```python
from build123d import *

# Parameters (mm, degrees)
SKETCH2_W           = 139.7
SKETCH2_H           = 88.9
BOSS_EXTRUDE1_DEPTH = 5.08
SKETCH3_R           = 1.905
BOSS_EXTRUDE2_DEPTH = 12.7
FILLET1_R           = 5.08
SKETCH4_W           = 25.4
SKETCH4_H           = 25.4
CUT_EXTRUDE1_DEPTH  = 5.08
FILLET2_R           = 5.08


with BuildPart() as part:
    # Sketch2 → Boss-Extrude1 (new body)
    with BuildSketch(Plane(origin=(0, 0, 0), x_dir=(0, 0, -1), z_dir=(1, 0, 0))):
        with Locations((0.114290462, 4.230322371)):
            Rectangle(SKETCH2_W, SKETCH2_H)
    extrude(amount=BOSS_EXTRUDE1_DEPTH)

    # Sketch3 → Boss-Extrude2 (add)
    with BuildSketch(Plane.ZY):
        with Locations((-62.344290462, 41.060322371)):
            Circle(SKETCH3_R)
        with Locations((-62.344290462, -32.599677629)):
            Circle(SKETCH3_R)
        with Locations((62.115709538, 41.060322371)):
            Circle(SKETCH3_R)
        with Locations((62.115709538, -32.599677629)):
            Circle(SKETCH3_R)
    extrude(amount=BOSS_EXTRUDE2_DEPTH)

    # Fillet1
    fillet1_edges = [part.edges().sort_by_distance(p)[0] for p in [
        (2.54, -40.219677629, 69.735709538),
        (2.54, 48.680322371, 69.735709538),
    ]]
    fillet(fillet1_edges, radius=FILLET1_R)

    # Sketch4 → Cut-Extrude1 (cut)
    with BuildSketch(Plane(origin=(5.08, 0, 0), x_dir=(0, 0, -1), z_dir=(1, 0, 0))):
        with Locations((31.864290462, -2.119677629)):
            Rectangle(SKETCH4_W, SKETCH4_H)
    extrude(amount=-CUT_EXTRUDE1_DEPTH, mode=Mode.SUBTRACT)

    # Fillet2
    fillet2_edges = [part.edges().sort_by_distance(p)[0] for p in [
        (2.54, 10.580322371, -44.564290462),
        (2.54, -14.819677629, -44.564290462),
        (2.54, -14.819677629, -19.164290462),
        (2.54, 10.580322371, -19.164290462),
    ]]
    fillet(fillet2_edges, radius=FILLET2_R)


solid = part.part
```
Work out the finished part from the listing and answer in its coordinate system (mm). A direction names the side the tool comes from. Give positions to 0.01 mm unless a question says otherwise; leave off trailing zeros. Loops run counter-clockwise (first coordinate to the right, second up) from the corner with the lowest first, then second, coordinate; pieces in that order, holes last. Notation, with made-up numbers: (0.25, 76.25) -> (19.25, 76.25) arc R16 cw to (19.25, 102.25) -> close; hole circle Ø1 at (-34.5, 40.25). An arc over 180 degrees is marked (long way). Write item = value, one per line. Start each with the question number.
(1) Find section A-A on y = -7.5. Give the vertices of the cut face in (x, z).
(2) Which of the six approach directions +Z, -Z, +X, -X, +Y, -Y give full straight-line access (tool end or side, diameter ignored) to faces 5 (the flat face through (-12.7, -33, -62)), 6 (the cylindrical face through (2.5, 9.13, -20.69)), 7 (the cylindrical face through (-6.261, 41.633, 63.933))?
(3) Find section C-C on z = -41. Give the vertices of the cut face in (x, y).
(4) Find the intervals of material crossed by probe 1 along Z at (x, y) = (3.5, -10); probe 2 along X at (y, z) = (-6.5, -15); probe 3 along Z at (x, y) = (-1.25, 42), in increasing order. Write a range as from..to.
(5) Find section D-D on z = 46. Give the vertices of the cut face in (x, y), and give its area (3 significant figures).
(6) Given pin 1 Ø5 at (y, z) = (10.5, 12) entering from -X, flat-ended and moving along its own axis, determine where the tip first touches the part or whether it passes through.
(7) Find section B-B on x = 2.25. Give the vertices of the cut face in (y, z).
(8) The mould has two halves that part along Z. Classify faces 1 (the cylindrical face through (2.58, -38.69, 68.29)), 2 (the flat face through (3, 4, -69.964)), 3 (the flat face through (-12.7, 41, 62)), 4 (the cylindrical face through (-6.261, -32.027, 63.933)): +Z half, -Z half, draft (parallel to the pull), parting line (faces both ways), or undercut.
From the geometry:
q1.outline = (0, -69.96) -> (5.08, -69.96) -> (5.08, -44.56) -> (0, -44.56) -> close; (0, -19.16) -> (5.08, -19.16) -> (5.08, 69.74) -> (0, 69.74) -> close
q2.face_5 = +Z, -Z, -X, +Y, -Y
q2.face_6 = +X, -X
q2.face_7 = -X
q3.outline = (0, -40.22) -> (5.08, -40.22) -> (5.08, -14.59) -> (0, -14.59) -> close; (0, 10.35) -> (5.08, 10.35) -> (5.08, 48.68) -> (0, 48.68) -> close
q4.probe_1 = -69.96..-44.56, -19.17..69.74
q4.probe_2 = 0..5.08
q4.probe_3 = -64..-60.69, 60.46..63.77
q5.outline = (0, -40.22) -> (5.08, -40.22) -> (5.08, 48.68) -> (0, 48.68) -> close
q5.area = 452 mm^2
q6.pin_1 = 0
q7.outline = (-40.22, -69.96) -> (48.68, -69.96) -> (48.68, 64.66) arc R5.08 ccw to (43.6, 69.74) -> (-35.14, 69.74) arc R5.08 ccw to (-40.22, 64.66) -> close; hole (-14.82, -39.48) arc R5.08 ccw to (-9.74, -44.56) -> (5.5, -44.56) arc R5.08 ccw to (10.58, -39.48) -> (10.58, -24.24) arc R5.08 ccw to (5.5, -19.16) -> (-9.74, -19.16) arc R5.08 ccw to (-14.82, -24.24) -> close
q8.face_1 = +Z half
q8.face_2 = -Z half
q8.face_3 = draft
q8.face_4 = undercut
